```python
from build123d import *

# Parameters (mm, degrees)
SKETCH1_R           = 3.25
BOSS_EXTRUDE1_DEPTH = 13.25
SKETCH2_W           = 23.25
SKETCH2_H           = 33.8
CUT_EXTRUDE1_DEPTH  = 12
CUT_EXTRUDE2_REACH  = 46.442
SKETCH3_R           = 2.625
SKETCH4_W           = 6.6
SKETCH4_H           = 1.7
CUT_EXTRUDE3_DEPTH  = 8
SKETCH5_W           = 23.25
SKETCH5_H           = 2
SKETCH5_H_2         = 1.8
BOSS_EXTRUDE2_DEPTH = 1.5
CUT_EXTRUDE4_REACH  = 38.105
SKETCH6_W           = 21.25
SKETCH6_H           = 23
SKETCH7_R           = 0.15
BOSS_EXTRUDE3_DEPTH = 13.25
BOSS_EXTRUDE4_START = 1
BOSS_EXTRUDE4_DEPTH = 1


with BuildPart() as part:
    # Sketch1 → Boss-Extrude1 (new body)
    with BuildSketch(Plane(origin=(0, 0, 0), x_dir=(1, 0, 0), z_dir=(0, 1, 0))):
        with BuildLine():
            Line((13, 27), (-13, 27))
            Line((-13, 27), (-13, 3.682729966))
            ThreePointArc((-13, 3.682729966), (-20.75, 0), (-13, -3.682729966))
            Line((-13, -3.682729966), (-13, -10))
            Line((-13, -10), (13, -10))
            Line((13, -10), (13, -3.682729966))
            ThreePointArc((13, -3.682729966), (20.75, 0), (13, 3.682729966))
            Line((13, 3.682729966), (13, 27))
        make_face()
        with Locations(Location((-16, 0, 0), (0, 0, 270))):
            Circle(SKETCH1_R, mode=Mode.SUBTRACT)
        with Locations(Location((16, 0, 0), (0, 0, 270))):
            Circle(SKETCH1_R, mode=Mode.SUBTRACT)
    extrude(amount=BOSS_EXTRUDE1_DEPTH)

    # Sketch2 → Cut-Extrude1 (cut)
    with BuildSketch(Plane(origin=(0, 13.25, 0), x_dir=(1, 0, 0), z_dir=(0, 1, 0))):
        with Locations((0, 10.1)):
            Rectangle(SKETCH2_W, SKETCH2_H)
    extrude(amount=-CUT_EXTRUDE1_DEPTH, mode=Mode.SUBTRACT)

    # Sketch3 → Cut-Extrude2 (cut, up to next)
    with BuildSketch(Plane.XY.offset(10), mode=Mode.PRIVATE) as cut_extrude2_sk1:
        with BuildLine():
            Line((3.9, 13.25), (3.9, 8.85))
            ThreePointArc((3.9, 8.85), (6.525, 11.475), (9.15, 8.85))
            Line((9.15, 8.85), (9.15, 13.25))
            Line((9.15, 13.25), (3.9, 13.25))
        make_face()
    cut_extrude2_tool1 = extrude(cut_extrude2_sk1.sketch, amount=-CUT_EXTRUDE2_REACH, mode=Mode.PRIVATE) & part.part
    # Sketch3 → Cut-Extrude2 (cut, up to next)
    with BuildSketch(Plane.XY.offset(10), mode=Mode.PRIVATE) as cut_extrude2_sk2:
        with Locations((6.525, 8.85)):
            Circle(SKETCH3_R)
    cut_extrude2_tool2 = extrude(cut_extrude2_sk2.sketch, amount=-CUT_EXTRUDE2_REACH, mode=Mode.PRIVATE) & part.part
    add(cut_extrude2_tool1.solids().sort_by_distance((6.525, 12.007435, 10))[0], mode=Mode.SUBTRACT)
    add(cut_extrude2_tool2.solids().sort_by_distance((6.525, 8.85, 10))[0], mode=Mode.SUBTRACT)

    # Sketch4 → Cut-Extrude3 (cut)
    with BuildSketch(Plane(origin=(0, 13.25, 0), x_dir=(1, 0, 0), z_dir=(0, 1, 0))):
        with Locations((6.525, -7.65)):
            Rectangle(SKETCH4_W, SKETCH4_H)
    extrude(amount=-CUT_EXTRUDE3_DEPTH, mode=Mode.SUBTRACT)

    # Sketch5 → Boss-Extrude2 (add)
    with BuildSketch(Plane(origin=(0, 1.25, 0), x_dir=(1, 0, 0), z_dir=(0, 1, 0))):
        with Locations((0, -0.8)):
            Rectangle(SKETCH5_W, SKETCH5_H)
        with Locations((0, 26.1)):
            Rectangle(SKETCH5_W, SKETCH5_H_2)
    extrude(amount=BOSS_EXTRUDE2_DEPTH)

    # Sketch6 → Cut-Extrude4 (cut, up to next)
    with BuildSketch(Plane(origin=(0, 1.25, 0), x_dir=(1, 0, 0), z_dir=(0, 1, 0)), mode=Mode.PRIVATE) as cut_extrude4_sk1:
        with Locations((0, 12.7)):
            Rectangle(SKETCH6_W, SKETCH6_H)
    cut_extrude4_tool1 = extrude(cut_extrude4_sk1.sketch, amount=-CUT_EXTRUDE4_REACH, mode=Mode.PRIVATE) & part.part
    add(cut_extrude4_tool1.solids().sort_by_distance((0, 1.25, -12.7))[0], mode=Mode.SUBTRACT)

    # Sketch7 → Boss-Extrude3 (add)
    with BuildSketch(Plane(origin=(0, 13.25, 0), x_dir=(1, 0, 0), z_dir=(0, 1, 0))):
        with Locations((-16, 3.25)):
            Circle(SKETCH7_R)
        with Locations((-19.25, 0)):
            Circle(SKETCH7_R)
        with Locations((-12.75, 0)):
            Circle(SKETCH7_R)
        with Locations((-16, -3.25)):
            Circle(SKETCH7_R)
        with Locations((16, -3.25)):
            Circle(SKETCH7_R)
        with Locations((12.75, 0)):
            Circle(SKETCH7_R)
        with Locations((19.25, 0)):
            Circle(SKETCH7_R)
        with Locations((16, 3.25)):
            Circle(SKETCH7_R)
    extrude(amount=-BOSS_EXTRUDE3_DEPTH)

    # Sketch8 → Boss-Extrude4 (add)
    with BuildSketch(Plane.XY.offset(10).offset(BOSS_EXTRUDE4_START)):
        with BuildLine():
            Line((3.9, 8.85), (3.9, 13.25))
            Line((3.9, 13.25), (-13, 13.25))
            Line((-13, 13.25), (-13, 0))
            Line((-13, 0), (13, 0))
            Line((13, 0), (13, 13.25))
            Line((13, 13.25), (9.15, 13.25))
            Line((9.15, 13.25), (9.15, 8.85))
            ThreePointArc((9.15, 8.85), (6.525, 6.225), (3.9, 8.85))
        make_face()
    extrude(amount=-BOSS_EXTRUDE4_DEPTH)


solid = part.part
```
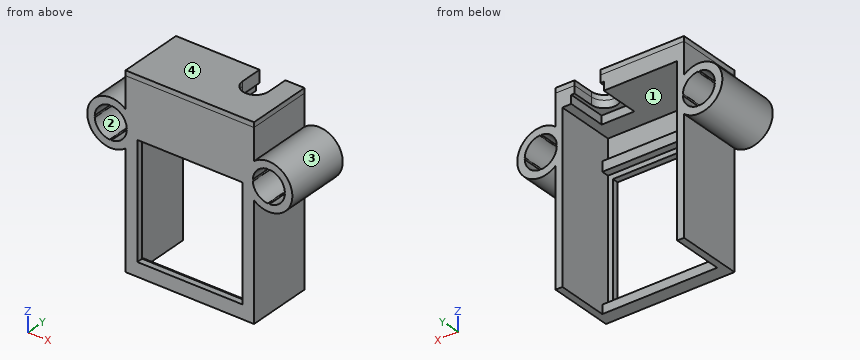
For this review, take the finished solid that the model builds, in its own axes (mm). Face numbers are marked on the shaded views. A direction names the side the tool comes from. Round coordinates to 2 decimals unless told otherwise and drop trailing zeros. Write each loop counter-clockwise with the first axis right and the second up, starting at its lowest first coordinate (ties: lowest second). Pieces come first, ordered by that corner, then holes. Notation, with made-up numbers: (40.5, 18) -> (65.5, 18) arc R20 cw to (65.5, 35) -> close; hole circle Ø11 at (68, 45). An arc over 180 degrees is marked (long way). Use one line per item in the form item = value.
1) Take a section at A-A, the plane y = 10. Count the separate pieces of the cut face and the enclosed holes in it, and give its area (3 significant figures).
Found:
separate_pieces = 2
enclosed_holes = 2
area = 236 mm2
2) Mouldability with a two-part tool opening along X and no side actions: class the marked faces 3 and 4 as +X half, -X half, draft (parallel to the pull), parting line (faces both ways), or undercut.
Found:
face_3 = undercut
face_4 = draft
3) Tool access review of the marked faces 1 and 2: name each direction out of +Z, -Z, +X, -X, +Y, -Y from which nothing blocks a thin tool from reaching the whole face with its end or side.
Found:
face_1 = +Y
face_2 = +Y, -Y
4) Take a section at B-B, the plane z = -6.5. Write out the cut boundary in (x, y) (3 decimals).
Found:
outline = (-13, 0) -> (-10.625, 0) -> (-10.625, 1.25) -> (-11.625, 1.25) -> (-11.625, 13.25) -> (-13, 13.25) -> close; (10.625, 0) -> (13, 0) -> (13, 13.25) -> (11.625, 13.25) -> (11.625, 1.25) -> (10.625, 1.25) -> close
5) To check wall thickness, follow L1, parallel to X at y = 4.25, z = -25 (3 decimals); L2, parallel to X at y = 12.5, z = 7.5 (3 decimals); L3, parallel to Z at x = -7, y = 9. State the ranges of each line that lie inside material, in increasing order. Write a range as from..to.
Found:
L1 = -13..-11.625, 11.625..13
L2 = -13..3.225, 9.825..13
L3 = 6.8..11
6) Take a section at C-C, the plane y = 3.5. Write out the cut boundary in (x, z) (3 decimals), and give its area (3 significant figures).
Found:
outline = (-13, -27) -> (-11.625, -27) -> (-11.625, 6.8) -> (11.625, 6.8) -> (11.625, -27) -> (13, -27) -> (13, -3.683) arc R4.75 ccw (long way) to (13, 3.683) -> (13, 11) -> (-13, 11) -> (-13, 3.683) arc R4.75 ccw (long way) to (-13, -3.683) -> close; hole (-19.247, -0.15) arc R3.25 ccw to (-16.15, -3.247) arc R0.15 cw to (-15.85, -3.247) arc R3.25 ccw to (-12.753, -0.15) arc R0.15 cw to (-12.753, 0.15) arc R3.25 ccw to (-15.85, 3.247) arc R0.15 cw to (-16.15, 3.247) arc R3.25 ccw to (-19.247, 0.15) arc R0.15 cw to start; hole (12.753, -0.15) arc R3.25 ccw to (15.85, -3.247) arc R0.15 cw to (16.15, -3.247) arc R3.25 ccw to (19.247, -0.15) arc R0.15 cw to (19.247, 0.15) arc R3.25 ccw to (16.15, 3.247) arc R0.15 cw to (15.85, 3.247) arc R3.25 ccw to (12.753, 0.15) arc R0.15 cw to start
area = 260 mm2
7) Clearance check with flat-ended pins moving along their axes: pin 1 (6 mm diameter, centred on y = 8.5, z = -10.5, fed in from -X); pin 2 (1.5 mm diameter, centred on y = 2, z = -2, fed in from -X); pin 3 (1 mm diameter, centred on y = 0.5, z = -18, fed in from +X). State where each tip first meets the part, or that it passes through.
Found:
pin_1 = -13
pin_2 = -20.58
pin_3 = 13
